from build123d import *

# Parameters (mm, degrees)
SKETCH1_W           = 80
SKETCH1_H           = 58
BOSS_EXTRUDE1_DEPTH = 13
SKETCH2_W           = 80
SKETCH2_H           = 17
BOSS_EXTRUDE2_DEPTH = 59
SKETCH3_W           = 80
SKETCH3_H           = 13
BOSS_EXTRUDE3_DEPTH = 41
SKETCH4_W           = 80
SKETCH4_H           = 17
BOSS_EXTRUDE4_DEPTH = 55.5
SKETCH5_W           = 10
SKETCH5_H           = 55.5
CUT_EXTRUDE1_DEPTH  = 55.5
SKETCH7_W           = 10
SKETCH7_H           = 55.5
CUT_EXTRUDE2_DEPTH  = 55.5
SKETCH8_R           = 30
BOSS_EXTRUDE5_DEPTH = 17
SKETCH9_R           = 7.5
CUT_EXTRUDE3_DEPTH  = 17
FILLET1_R           = 10
FILLET2_R           = 10
CUT_EXTRUDE4_DEPTH  = 17
CUT_EXTRUDE5_DEPTH  = 17
SKETCH12_R          = 6
CUT_EXTRUDE6_DEPTH  = 17
SKETCH13_R          = 6
CUT_EXTRUDE7_DEPTH  = 17


with BuildPart() as part:
    # Sketch1 → Boss-Extrude1 (new body)
    with BuildSketch(Plane(origin=(0, 0, 0), x_dir=(1, 0, 0), z_dir=(0, 1, 0))):
        Rectangle(SKETCH1_W, SKETCH1_H)
    extrude(amount=BOSS_EXTRUDE1_DEPTH)

    # Sketch2 → Boss-Extrude2 (add)
    with BuildSketch(Plane(origin=(0, 13, 0), x_dir=(1, 0, 0), z_dir=(0, 1, 0))):
        with Locations((0, 20.5)):
            Rectangle(SKETCH2_W, SKETCH2_H)
    extrude(amount=BOSS_EXTRUDE2_DEPTH)

    # Sketch3 → Boss-Extrude3 (add)
    with BuildSketch(Plane.XY.offset(-12)):
        with Locations((0, 65.5)):
            Rectangle(SKETCH3_W, SKETCH3_H)
    extrude(amount=BOSS_EXTRUDE3_DEPTH)

    # Sketch4 → Boss-Extrude4 (add)
    with BuildSketch(Plane(origin=(0, 72, 0), x_dir=(1, 0, 0), z_dir=(0, 1, 0))):
        with Locations((0, 20.5)):
            Rectangle(SKETCH4_W, SKETCH4_H)
    extrude(amount=BOSS_EXTRUDE4_DEPTH)

    # Sketch5 → Cut-Extrude1 (cut)
    with BuildSketch(Plane.XY.offset(-12)):
        with Locations((-35, 99.75)):
            Rectangle(SKETCH5_W, SKETCH5_H)
    extrude(amount=-CUT_EXTRUDE1_DEPTH, mode=Mode.SUBTRACT)

    # Sketch7 → Cut-Extrude2 (cut)
    with BuildSketch(Plane.XY.offset(-12)):
        with Locations((35, 99.75)):
            Rectangle(SKETCH7_W, SKETCH7_H)
    extrude(amount=-CUT_EXTRUDE2_DEPTH, mode=Mode.SUBTRACT)

    # Sketch8 → Boss-Extrude5 (add)
    with BuildSketch(Plane.XY.offset(-12)):
        with Locations((0, 127.5)):
            Circle(SKETCH8_R)
    extrude(amount=-BOSS_EXTRUDE5_DEPTH)

    # Sketch9 → Cut-Extrude3 (cut)
    with BuildSketch(Plane.XY.offset(-12)):
        with Locations((0, 127.5)):
            Circle(SKETCH9_R)
    extrude(amount=-CUT_EXTRUDE3_DEPTH, mode=Mode.SUBTRACT)

    # Fillet1
    fillet1_edges = [part.edges().sort_by_distance(p)[0] for p in [
        (-30, 72, -20.5),
    ]]
    fillet(fillet1_edges, radius=FILLET1_R - 0.0001)  # a hair under: the kernel refuses the full size

    # Fillet2
    fillet2_edges = [part.edges().sort_by_distance(p)[0] for p in [
        (30, 72, -20.5),
    ]]
    fillet(fillet2_edges, radius=FILLET2_R - 0.0001)  # a hair under: the kernel refuses the full size

    # Sketch10 → Cut-Extrude4 (cut)
    with BuildSketch(Plane(origin=(0, 13, 0), x_dir=(1, 0, 0), z_dir=(0, 1, 0))):
        with BuildLine():
            Line((-26, -9.5), (26, -9.5))
            ThreePointArc((26, -9.5), (32.5, -16), (26, -22.5))
            Line((26, -22.5), (-26, -22.5))
            ThreePointArc((-26, -22.5), (-32.5, -16), (-26, -9.5))
        make_face()
    extrude(amount=-CUT_EXTRUDE4_DEPTH, mode=Mode.SUBTRACT)

    # Sketch11 → Cut-Extrude5 (cut)
    with BuildSketch(Plane(origin=(0, 72, 0), x_dir=(1, 0, 0), z_dir=(0, 1, 0))):
        with BuildLine():
            Line((-26, -9.5), (26, -9.5))
            ThreePointArc((26, -9.5), (32.5, -16), (26, -22.5))
            Line((26, -22.5), (-26, -22.5))
            ThreePointArc((-26, -22.5), (-32.5, -16), (-26, -9.5))
        make_face()
    extrude(amount=-CUT_EXTRUDE5_DEPTH, mode=Mode.SUBTRACT)

    # Sketch12 → Cut-Extrude6 (cut)
    with BuildSketch(Plane.XY.offset(-12)):
        with Locations((-21.5, 30)):
            Circle(SKETCH12_R)
    extrude(amount=-CUT_EXTRUDE6_DEPTH, mode=Mode.SUBTRACT)

    # Sketch13 → Cut-Extrude7 (cut)
    with BuildSketch(Plane.XY.offset(-12)):
        with Locations((21.5, 30)):
            Circle(SKETCH13_R)
    extrude(amount=-CUT_EXTRUDE7_DEPTH, mode=Mode.SUBTRACT)


solid = part.part
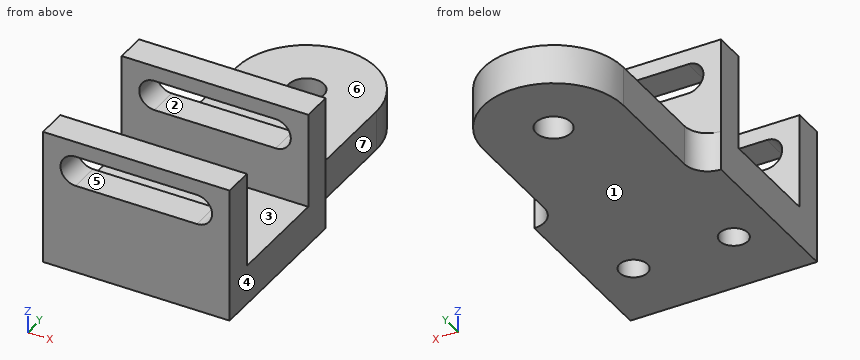
The model under review builds one solid part; all positions refer to its coordinate system, in mm. Face numbers are marked on the shaded views. A direction names the side the tool comes from. Coordinates: 2 decimals unless noted, no trailing zeros. Loops run counter-clockwise (first coordinate to the right, second up) from the corner with the lowest first, then second, coordinate; pieces in that order, holes last. Notation, with made-up numbers: M 15.5,-1.75 L 49.5,-1.75 A27 ccw 49.5,16.25 Z; hole C 66.5,-38.5 d6. An arc over 180 degrees is marked long. Put each result on its own line as item: value. Start each with the question number.
Q1. The part is to be moulded in two halves that separate along Z. For the marked faces 1, 2, 3 and 4, say which applies: +Z half, -Z half, draft (parallel to the pull), parting line (faces both ways), or undercut.
Q2. Clearance check with flat-ended pins moving along their axes: pin 1 (3 mm diameter, centred on x = 7, z = -18.5, fed in from -Y); pin 2 (8.5 mm diameter, centred on y = 95.5, z = -21.5, fed in from +X); pin 3 (18.5 mm diameter, centred on y = 103, z = -21, fed in from -X); pin 4 (23 mm diameter, centred on x = 3.5, y = 33.5, fed in from +Z). State where each tip first meets the part, or that it passes through.
Q3. Add section D-D (z = 16). Write out the cut boundary in (x, y), and give its area (3 significant figures).
Q4. Add section A-A (x = 0). Write out the cut boundary in (y, z).
Q5. Wall thickness on line 1 (Z direction, x = -2, y = 62); line 2 (Y direction, x = 4.5, z = 8); line 3 (X direction, y = 105, z = -16): over which ranges is each line inside the solid? List them lowest first.
Q6. For the marked faces 5, 6 and 7, list the 3-axis set-ups (+Z, -Z, +X, -X, +Y, -Y) from which the entire face can be reached by the end or side of a thin tool; tool diameter is ignored.
Q7. Add section B-B (z = -20). Count the separate pieces of the cut face and the enclosed holes in it, and give its area (3 significant figures).
Q8. Add section C-C (y = 30). Write out the cut boundary in (x, z), and give its area (3 significant figures).
Answers:
1. face 1: -Z half
1. face 2: undercut
1. face 3: +Z half
1. face 4: draft
2. pin 1: stops at y = 0
2. pin 2: stops at x = 30
2. pin 3: stops at x = -30
2. pin 4: stops at z = -12
3. outline: M -40,0 L -32.5,0 L -32.5,13 L -40,13 Z; M -40,59 L -32.5,59 L -32.5,72 L -40,72 Z; M 32.5,0 L 40,0 L 40,13 L 32.5,13 Z; M 32.5,59 L 40,59 L 40,72 L 32.5,72 Z
3. area: 390 mm^2
4. outline: M 0,-29 L 120,-29 L 120,-12 L 72,-12 L 72,9.5 L 59,9.5 L 59,-12 L 13,-12 L 13,9.5 L 0,9.5 Z; M 0,22.5 L 13,22.5 L 13,29 L 0,29 Z; M 59,22.5 L 72,22.5 L 72,29 L 59,29 Z; M 135,-29 L 157.5,-29 L 157.5,-12 L 135,-12 Z
5. line 1: z = -29 to 9.5, 22.5 to 29
5. line 2: y = 0 to 13, 59 to 72
5. line 3: x = -30 to 30
6. face 5: +Y, -Y
6. face 6: +Z, +X, -X, +Y
6. face 7: +Z, -Z, +X, +Y
7. separate pieces: 1
7. enclosed holes: 3
7. area: 10,100 mm^2
8. outline: M -40,-29 L -27.5,-29 L -27.5,-12 L -40,-12 Z; M -15.5,-29 L 15.5,-29 L 15.5,-12 L -15.5,-12 Z; M 27.5,-29 L 40,-29 L 40,-12 L 27.5,-12 Z
8. area: 952 mm^2
